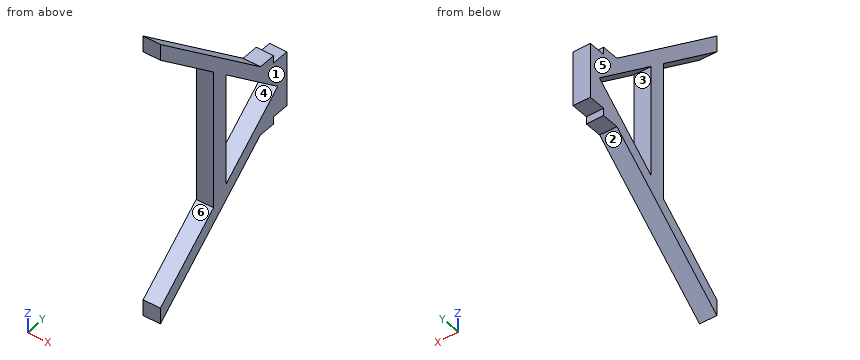
```python
from build123d import *

# Parameters (mm, degrees)
BOSS_EXTRUDE2_DEPTH = 3.175


with BuildPart() as part:
    # Sketch1 → Boss-Extrude2 (new body)
    with BuildSketch(Plane(origin=(0, 0, 0), x_dir=(0, 0, -1), z_dir=(1, 0, 0))):
        Polygon((0.727545577, -5.496236961), (-19.379740188, -29.459167008), (-16.379740188, -29.459167008), (-5.695435338, -16.726108319), (20.150526491, -16.726108319), (30.834831341, -29.459167008), (33.834831341, -29.459167008), (13.727545577, -5.496236961), (13.727545577, -2.321236961), (12.352545577, -2.321236961), (12.352545577, 0.853763039), (2.102545577, 0.853763039), (2.102545577, -2.321236961), (0.727545577, -2.321236961), align=None)
        Polygon((7.227545577, -1.325099387), (17.633227598, -13.726108319), (-3.178136444, -13.726108319), align=None, mode=Mode.SUBTRACT)
    extrude(amount=BOSS_EXTRUDE2_DEPTH)


solid = part.part
```
Input: part model. Units: mm. Frame: model coordinates. Face numbers are marked on the shaded views. A direction names the side the tool comes from. Round coordinates to 2 decimals unless told otherwise and drop trailing zeros. Loops run counter-clockwise (first coordinate to the right, second up) from the corner with the lowest first, then second, coordinate; pieces in that order, holes last. Notation, with made-up numbers: (63, 42) - (105, 42) arc R15 ccw to (105, 66) - close; hole circle Ø8 at (54.25, -12). An arc over 180 degrees is marked (long way). One line per item, written item: value. Start each with the question number.
(1) Section D-D, the plane z = 10. Return loops of the section in (x, y) (3 decimals).
(2) Access query for the marked faces 5 and 6. Directions: +Z, -Z, +X, -X, +Y, -Y. A direction counts if a zero-diameter tool reaches every point of the face in a straight line with its end or side. Return the directions, or none.
(3) Section C-C, the plane y = -6. Return loops of the section in (x, z) (3 decimals), plus the area to 4 significant figures.
(4) Ray query, line 1 (Z direction, x = 2.9, y = -2); line 2 (Z direction, x = 0.45, y = -23.5); line 3 (Y direction, x = 2.2, z = 3). Return the intervals inside material, ascending. Write a range as [from, to].
(5) Contact query for flat-ended pins moving along their axis: P1, Ø4, axis at y = -19.5, z = -12, coming from the +X side; P2, Ø1.6, axis at x = 2, z = -2, coming from the -Y side; P3, Ø1, axis at x = 1.5, y = -3.5, coming from the +Z side. Output: stop coordinate, or through.
(6) Section B-B, the plane z = -6.5. Return loops of the section in (x, y) (3 decimals).
(7) Draft query along Z for the marked faces 1, 2, 3 and 4. Return one class per face: +Z half, -Z half, draft (parallel to the pull), parting line (faces both ways), or undercut.
(8) Section A-A, the plane x = 1.25. Return loops of the section in (y, z), plus the area to 3 significant figures.
Results below:
1. outline: (0, -21.856) - (3.175, -21.856) - (3.175, -18.281) - (0, -18.281) - close
2. face 5: +Z, -Z, -X, +Y, -Y
2. face 6: +X, -X, -Y
3. outline: (0, -14.15) - (3.175, -14.15) - (3.175, -11.15) - (0, -11.15) - close; (0, -3.305) - (3.175, -3.305) - (3.175, -0.305) - (0, -0.305) - close
3. area: 19.05 mm^2
4. line 1: [-12.35, -7.79], [-6.66, -2.1]
4. line 2: [-28.83, -25.83], [11.38, 14.38]
4. line 3: [-16.73, -13.73], [-13.51, -9.94]
5. P1: through
5. P2: y = -16.73
5. P3: z = -0.73
6. outline: (0, -16.726) - (3.175, -16.726) - (3.175, -13.726) - (0, -13.726) - close; (0, -2.192) - (3.175, -2.192) - (3.175, 0.854) - (0, 0.854) - close
7. face 1: draft
7. face 2: -Z half
7. face 3: undercut
7. face 4: undercut
8. outline: (-29.46, -33.83) - (-5.5, -13.73) - (-2.32, -13.73) - (-2.32, -12.35) - (0.85, -12.35) - (0.85, -2.1) - (-2.32, -2.1) - (-2.32, -0.73) - (-5.5, -0.73) - (-29.46, 19.38) - (-29.46, 16.38) - (-16.73, 5.7) - (-16.73, -20.15) - (-29.46, -30.83) - close; hole (-13.73, -17.63) - (-1.33, -7.23) - (-13.73, 3.18) - close
8. area: 273 mm^2
